Work out the finished part from the listing and answer in its coordinate system (mm). A direction names the side the tool comes from. Round coordinates to 2 decimals unless told otherwise and drop trailing zeros. Loops run counter-clockwise (first coordinate to the right, second up) from the corner with the lowest first, then second, coordinate; pieces in that order, holes last.
from build123d import *

# Parameters (mm, degrees)
F0_R     = 9.525
F1_DEPTH = 25.4
F3_DEPTH = 25.401
F4_DEPTH = 11.0998
F6_DEPTH = 9.525


with BuildPart() as f1:
    # F0 (on Front) → F1 (new body)
    with BuildSketch(Plane.XZ):
        Circle(F0_R)
    extrude(amount=F1_DEPTH)

    # F2 (on face) → F3 (cut, through all)
    with BuildSketch(Plane.XZ.offset(25.4)):
        with BuildLine():
            ThreePointArc((4.7625, 0), (3.367596, 3.367596), (0, 4.7625))
            ThreePointArc((0, 4.7625), (-3.367596, 3.367596), (-4.7625, 0))
            ThreePointArc((-4.7625, 0), (-3.367596, -3.367596), (0, -4.7625))
            ThreePointArc((0, -4.7625), (3.367596, -3.367596), (4.7625, 0))
        make_face()
    extrude(amount=-F3_DEPTH, mode=Mode.SUBTRACT)

    # F2 (on face) → F4 (cut)
    with BuildSketch(Plane.XZ.offset(25.4)):
        with BuildLine():
            Line((4.7625, 0), (4.7625, 4.7625))
            Line((4.7625, 4.7625), (0, 4.7625))
            ThreePointArc((0, 4.7625), (3.367596, 3.367596), (4.7625, 0))
        make_face()
        with BuildLine():
            ThreePointArc((-4.7625, 0), (-3.367596, 3.367596), (0, 4.7625))
            Line((0, 4.7625), (-4.7625, 4.7625))
            Line((-4.7625, 4.7625), (-4.7625, 0))
        make_face()
        with BuildLine():
            Line((4.7625, -4.7625), (4.7625, 0))
            ThreePointArc((4.7625, 0), (3.367596, -3.367596), (0, -4.7625))
            Line((0, -4.7625), (4.7625, -4.7625))
        make_face()
        with BuildLine():
            ThreePointArc((0, -4.7625), (-3.367596, -3.367596), (-4.7625, 0))
            Line((-4.7625, 0), (-4.7625, -4.7625))
            Line((-4.7625, -4.7625), (0, -4.7625))
        make_face()
    extrude(amount=-F4_DEPTH, mode=Mode.SUBTRACT)

    # F5 (on face) → F6 (cut)
    with BuildSketch(Plane(origin=(0, 0, 0), x_dir=(-1, 0, 0), z_dir=(0, 1, 0))):
        Polygon((3.932339, 6.811012), (-3.932339, 6.811012), (-7.864679, 0), (-3.932339, -6.811012), (3.932339, -6.811012), (7.864679, 0), align=None)
    extrude(amount=-F6_DEPTH, mode=Mode.SUBTRACT)


solid = f1.part
Item 1: Straight lines are drawn through the part: line 1 (Z direction, x = -2, y = -2); line 2 (X direction, y = -20, z = -2); line 3 (Y direction, x = -5.5, z = 1) (3 decimals). For each, find the intervals that lie inside material, in ascending order.
Item 2: Each of these flat-tipped pins is pushed along its axis until it touches: P1, Ø5, axis at y = -20.5, z = -1, coming from the +X side (3 decimals); P2, Ø6, axis at x = 3.5, y = -10.5, coming from the -Z side; P3, Ø1, axis at x = -3.5, y = -3, coming from the +Z side; P4, Ø1, axis at x = 2.5, y = -6, coming from the -Z side. Where does it stop, or does it pass through?
Item 3: Section B-B, the plane z = -2.75 is taken. Give the vertices of the cut face in (x, y) (1 decimal), plus the area to 3 significant figures.
Item 4: For faces 5 (the face through (4, -14.3, 4)), 6 (the face through (5.871, -4.696, 3.453)), 7 (the face through (0, -25.4, -6)), determine the directions among +Z, -Z, +X, -X, +Y, -Y from which every point of the face is accessible in a straight line to the end or side of a thin tool.
Item 5: Section D-D, the plane x = 5.5 is taken. Give the vertices of the cut face in (y, z) (3 decimals), plus the area to 3 significant figures.
Item 6: Section A-A, the plane x = -3.5 is taken. Give the vertices of the cut face in (y, z) (1 decimal).
Item 7: Determine the mould class of faces 1 (the face through (-5.9, -4.7, 3.4)), 2 (the face through (4, -14.3, -4)), 3 (the face through (1, 0, -7)), 4 (the face through (-7.559, -12.522, -5.796)) for opening direction Z: pulls with the +Z half, pulls with the -Z half, needs draft (parallel to the pull), parting line crosses it, or undercut.
Answer below:
1. line 1: z = -9.31 to -6.81, 6.81 to 9.31
1. line 2: x = -9.31 to -4.76, 4.76 to 9.31
1. line 3: y = -25.4 to -9.525
2. P1: stops at x = 9.525
2. P2: stops at z = -9.51
2. P3: stops at z = 9.04
2. P4: stops at z = -9.31
3. outline: (-9.1, -25.4) - (-4.8, -25.4) - (-4.8, -14.3) - (-3.9, -14.3) - (-3.9, -9.5) - (-6.3, -9.5) - (-6.3, 0) - (-9.1, 0) - close; (3.9, -14.3) - (4.8, -14.3) - (4.8, -25.4) - (9.1, -25.4) - (9.1, 0) - (6.3, 0) - (6.3, -9.5) - (3.9, -9.5) - close
3. area: 201 mm2
4. face 5: -Y
4. face 6: +Y
4. face 7: +Z, -Z, +X, -X, -Y
5. outline: (-25.4, -7.777) - (0, -7.777) - (0, -4.096) - (-9.525, -4.096) - (-9.525, 4.096) - (0, 4.096) - (0, 7.777) - (-25.4, 7.777) - close
5. area: 317 mm2
6. outline: (-25.4, -8.9) - (0, -8.9) - (0, -6.8) - (-9.5, -6.8) - (-9.5, -3.2) - (-14.3, -3.2) - (-14.3, -4.8) - (-25.4, -4.8) - close; (-25.4, 4.8) - (-14.3, 4.8) - (-14.3, 3.2) - (-9.5, 3.2) - (-9.5, 6.8) - (0, 6.8) - (0, 8.9) - (-25.4, 8.9) - close
7. face 1: undercut
7. face 2: undercut
7. face 3: needs draft
7. face 4: parting line crosses it
